```python
from build123d import *

# Parameters (mm, degrees)
F0_W             = 609.6
F0_H             = 6.35
F1_DEPTH         = 25.4
F2_W             = 6.35
F2_H             = 609.6
F3_DEPTH         = 25.4
F4_W             = 6.35
F4_H             = 31.75
F5_DEPTH         = 609.6
F6_W             = 25.4
F6_H             = 6.35
F7_DEPTH         = 590.55
F12_D            = 6.35
F12_DEPTH        = 6.35
F12_TIP          = 1.9077324654
F13_D            = 6.35
F13_DEPTH        = 6.35
F13_TIP          = 1.9077324654
F13_ON_F10_D     = 6.35
F13_ON_F10_DEPTH = 6.35
F13_ON_F10_TIP   = 1.9077324654
F13_ON_F9_D      = 6.35
F13_ON_F9_DEPTH  = 6.35
F13_ON_F9_TIP    = 1.9077324654


with BuildPart() as f1:
    # F0 (on Right) → F1 (new body)
    with BuildSketch(Plane.YZ):
        with Locations((257.997608562, 58.7304569781)):
            Rectangle(F0_W, F0_H)
    extrude(amount=F1_DEPTH)

    # F2 (on face) → F3 (join)
    with BuildSketch(Plane(origin=(0, 0, 55.5554569781), x_dir=(1, 0, 0), z_dir=(0, 0, -1))):
        with Locations((3.175, -257.997608562)):
            Rectangle(F2_W, F2_H)
    extrude(amount=F3_DEPTH)

    # F4 (on face) → F5 (join)
    with BuildSketch(Plane.YZ.offset(6.35)):
        with Locations((559.622608562, 46.0304569781)):
            Rectangle(F4_W, F4_H)
    extrude(amount=F5_DEPTH)

    # F6 (on face) → F7 (join)
    with BuildSketch(Plane.YZ.offset(25.4)):
        with Locations((543.747608562, 58.7304569781)):
            Rectangle(F6_W, F6_H)
    extrude(amount=F7_DEPTH)

    # F12
    with Locations(Plane.XY.offset(61.9054569781)):
        with Locations((12.7, 359.597608562), (12.7, 153.222608562)):
            Hole(F12_D / 2, depth=F12_DEPTH)
            with Locations((0, 0, -(F12_DEPTH + F12_TIP / 2))):  # 118° drill point
                Cone(0, F12_D / 2, F12_TIP, mode=Mode.SUBTRACT)

    # F13
    with Locations(Plane(origin=(0, 0, 0), x_dir=(0, -1, 0), z_dir=(-1, 0, 0))):
        with Locations((-359.597608562, 49.2054569781), (-156.397608562, 49.2054569781)):
            Hole(F13_D / 2, depth=F13_DEPTH)
            with Locations((0, 0, -(F13_DEPTH + F13_TIP / 2))):  # 118° drill point
                Cone(0, F13_D / 2, F13_TIP, mode=Mode.SUBTRACT)

    # F13 on F10
    with Locations(Plane(origin=(0, 562.797608562, 0), x_dir=(-1, 0, 0), z_dir=(0, 1, 0))):
        with Locations((-203.2, 49.2054569781), (-406.4, 49.2054569781)):
            Hole(F13_ON_F10_D / 2, depth=F13_ON_F10_DEPTH)
            with Locations((0, 0, -(F13_ON_F10_DEPTH + F13_ON_F10_TIP / 2))):  # 118° drill point
                Cone(0, F13_ON_F10_D / 2, F13_ON_F10_TIP, mode=Mode.SUBTRACT)

    # F13 on F9
    with Locations(Plane.XY.offset(61.9054569781)):
        with Locations((406.4, 550.097608562), (203.2, 550.097608562)):
            Hole(F13_ON_F9_D / 2, depth=F13_ON_F9_DEPTH)
            with Locations((0, 0, -(F13_ON_F9_DEPTH + F13_ON_F9_TIP / 2))):  # 118° drill point
                Cone(0, F13_ON_F9_D / 2, F13_ON_F9_TIP, mode=Mode.SUBTRACT)


solid = f1.part
```
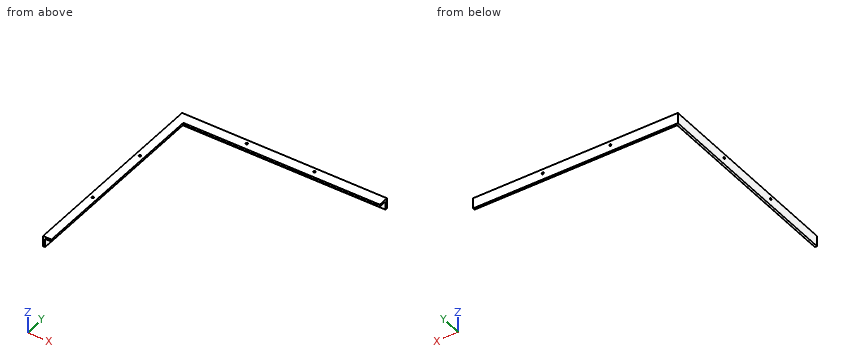
Work out the finished part from the listing and answer in its coordinate system (mm). Round coordinates to 2 decimals unless told otherwise and drop trailing zeros. Loops run counter-clockwise (first coordinate to the right, second up) from the corner with the lowest first, then second, coordinate; pieces in that order, holes last. Notation, with made-up numbers: (87, 47.5) -> (93, 47.5) arc R20 ccw to (93, 74.5) -> close; hole circle Ø11 at (50, 65.25). An arc over 180 degrees is marked (long way). Write each question's results on one line, items separated by ' | '. Start each with the question number.
1. Find the intervals of material crossed by probe 1 along Y at (x, z) = (12, 60); probe 2 along Y at (x, z) = (123, 35.5); probe 3 along X at (y, z) = (95.5, 48), in increasing order. Write a range as from..to.
2. Section B-B (z = 37.5) is taken. Determine the outline of the cut face in (x, y).
3. Section A-A (x = 570) is taken. Determine the outline of the cut face in (y, z).
4. Given pin 1 Ø1.5 at (y, z) = (144, 53.5) entering from +X; pin 2 Ø1 at (x, z) = (490, 34) entering from -Y; pin 3 Ø7 at (x, z) = (342, 59) entering from -Y; pin 4 Ø3 at (y, z) = (321.5, 36.5) entering from -X, each flat-ended and moving along its own axis, determine where each tip first touches the part or whether it passes through.
Evaluation:
1) probe 1: y = -46.8..150.13, 156.32..356.5, 362.69..562.8 | probe 2: y = 556.45..562.8 | probe 3: x = 0..6.35
2) outline: (0, -46.8) -> (6.35, -46.8) -> (6.35, 556.45) -> (615.95, 556.45) -> (615.95, 562.8) -> (0, 562.8) -> close
3) outline: (531.05, 55.56) -> (556.45, 55.56) -> (556.45, 30.16) -> (562.8, 30.16) -> (562.8, 61.91) -> (531.05, 61.91) -> close
4) pin 1: stops at x = 6.35 | pin 2: stops at y = 556.45 | pin 3: stops at y = 531.05 | pin 4: stops at x = 0
